The model under review builds one solid part; all positions refer to its coordinate system, in mm. A direction names the side the tool comes from. Round coordinates to 2 decimals unless told otherwise and drop trailing zeros. Loops run counter-clockwise (first coordinate to the right, second up) from the corner with the lowest first, then second, coordinate; pieces in that order, holes last. Notation, with made-up numbers: M 55.25,79.5 L 112.25,79.5 A28 cw 112.25,110.5 Z; hole C 17.25,64.5 d6. An arc over 180 degrees is marked long. One line per question, with ' | ' between items.
from build123d import *

# Parameters (mm, degrees)
FILETE2_R = 0.5
FILETE4_R = 6


with BuildPart() as part:
    # Esboço1 → Revolução1 (revolve)
    with BuildSketch(Plane.XY, mode=Mode.PRIVATE) as revolu_o1_sk:
        Polygon((0, 0), (92, 0), (92, 7), (82, 7), (82, 6.5), (80, 6.5), (80, 7), (48, 7), (43, 4.8), (13, 4.8), (6, 3.25), (6, 1), (0, 1), align=None)
    revolve(revolu_o1_sk.sketch.rotate(Axis((0, 0, 0), (1, 0, 0)), 90), axis=Axis((0, 0, 0), (1, 0, 0)))

    # Filete2
    filete2_edges = [part.edges().sort_by_distance(p)[0] for p in [
        (6, 0, -3.25),
    ]]
    fillet(filete2_edges, radius=FILETE2_R)

    # Filete4
    filete4_edges = [part.edges().sort_by_distance(p)[0] for p in [
        (13, 0, -4.8),
    ]]
    fillet(filete4_edges, radius=FILETE4_R)


solid = part.part
1) Insertion check: P1, Ø8, axis at x = 47.5, y = -5, coming from the +Z side; P2, Ø6, axis at y = 0.5, z = 4.5, coming from the -X side; P3, Ø2, axis at x = 82.5, z = 3, coming from the -Y side. Each pin has a flat end and moves straight along its axis. Give the tip position at first contact, or say it passes through.
Output values:
P1: stops at z = 6.92 | P2: stops at x = 6 | P3: stops at y = -6.71
2) Mouldability with a two-part tool opening along X and no side actions: class faces 1 (the cylindrical face through (3, 1, 0)), 2 (the cylindrical face through (80.986, 3.955, -5.158)), 3 (the flat face through (0, 0, 0)) as +X half, -X half, draft (parallel to the pull), parting line (faces both ways), or undercut.
Output values:
face 1: draft | face 2: undercut | face 3: -X half
3) For line 1 (X direction, y = 5.25, z = 4); line 2 (X direction, y = -1, z = 1); line 3 (X direction, y = 6.25, z = -2) (3 decimals), list the stretches that pass through material, from the lowest coordinate up.
Output values:
line 1: x = 47.09 to 80, 82 to 92 | line 2: x = 6 to 92 | line 3: x = 47.005 to 80, 82 to 92
4) Add section A-A on x = 61.5. State the section outline as (y, z) points.
Output values:
outline: C 0,0 d14
5) Machinability: for faces 4 (the flat face through (92, 0, 0)), 5 (the flat face through (6, 1.2, 0)), which of the approach directions +Z, -Z, +X, -X, +Y, -Y give a long, thin tool a straight path to every point of the face, cutting with its end or side? Answer none if there is none.
Output values:
face 4: +Z, -Z, +X, +Y, -Y | face 5: -X
